Input: part model. Units: mm. Frame: model coordinates. A direction names the side the tool comes from. Give positions to 0.01 mm unless a question says otherwise; leave off trailing zeros. Write each loop counter-clockwise with the first axis right and the second up, starting at its lowest first coordinate (ties: lowest second). Pieces come first, ordered by that corner, then holes.
Autodesk Inventor part; units mm, degrees
ref_plane "Work Plane1" through (72.225, 0, 0) normal (1, 0, 0) x (0, 0, -1)
ref_plane "YZ Plane" through (0, 0, 0) normal (1, 0, 0) x (0, 1, 0)
ref_plane "XZ Plane" through (0, 0, 0) normal (0, 1, 0) x (-1, 0, 0)
sketch "Sketch1" plane through (0, 0, 0) normal (1, 0, 0) x (0, 1, 0)
  circle A0 centre (0, 0) radius 10
  arc A1 (-9.7398, 12.694) -> (5.3275, -15.087) centre (0, 0) ccw
  line L0 (0, 0) -> (0, 61.6) construction
  line L1 (0, 0) -> (54, 0) construction
  line L2 (0, 61.6) -> (54, 61.6) construction
  line L3 (54, 0) -> (54, 61.6) construction
  line L4 (54, 61.6) -> (54, 2.1)
  line L5 (54, 61.6) -> (-9.7398, 12.694)
  line L6 (54, 2.1) -> (5.3275, -15.087)
  dimension "d0" = 20
  dimension "d2" = 32
  dimension "d3" = 61.6
  dimension "d4" = 54
  dimension "d5" = 59.5
extrude "Extrusion1" add sketch "Sketch1" along normal blind 144.45
sketch "Sketch2" plane through (0, 0, 0) normal (0, 0, 1) x (1, 0, 0)
  line L0 (0, 54) -> (144.45, 54)
  line L1 (0, -9.7398) -> (0, 54)
  line L2 (0, -9.7398) -> (144.45, -9.7398)
  line L3 (144.45, 54) -> (144.45, -9.7398)
  line L4 (0, 54) -> (144.45, 54)
  line L5 (72.225, 54) -> (72.225, -21.6932)
  line L6 (39.225, 48) -> (105.225, 48)
  line L7 (105.225, 48) -> (105.225, -39.8615)
  line L8 (105.225, -39.8615) -> (39.225, -39.8615)
  line L9 (39.225, -39.8615) -> (39.225, 48)
  line L10 (72.225, 48) -> (72.225, -39.8615)
  point P0 (0, 0)
  dimension "d8" = 66
  dimension "d10" = 6
extrude "Extrusion2" cut sketch "Sketch2" along normal mid plane 144.45 contours L6 L7 L2 L5 | L5 L2 L9 L6 | L2 L5 L10 L8 L9 | L2 L7 L8 L10 L5
ref_plane "Work Plane1" through (72.225, 0, 0) normal (1, 0, 0) x (0, 0, -1)
sketch "Sketch3" plane through (0, 0, 0) normal (0, 0, 1) x (1, 0, 0)
  line L0 (0, 54) -> (144.45, 54)
  line L1 (144.45, 54) -> (144.45, -9.7398)
  line L2 (105.225, 48) -> (105.225, -9.7398)
  line L3 (105.225, -9.7398) -> (144.45, -9.7398)
  line L4 (144.45, 54) -> (144.45, -9.7398)
  line L5 (0, 54) -> (144.45, 54)
  line L6 (0, -9.7398) -> (0, 54)
  line L7 (0, -9.7398) -> (39.225, -9.7398)
  line L8 (39.225, -9.7398) -> (39.225, 48)
  line L9 (39.225, 48) -> (105.225, 48)
  line L10 (144.45, 48) -> (109.925, 48)
  line L11 (109.925, 48) -> (109.925, -25.7164)
  line L12 (109.925, -25.7164) -> (144.45, -25.7164)
  line L13 (144.45, -25.7164) -> (144.45, 48)
  line L14 (39.225, 48) -> (105.225, 48)
  point P0 (0, 0)
  dimension "d14" = 34.525
extrude "Extrusion3" cut sketch "Sketch3" along normal through all both and the other way through all contours L1 L3 L11 L10 | L13 L12 L11 L3
mirror "Mirror1" about plane through (72.225, 0, 0) normal (1, 0, 0) of "Extrusion3"
move or copy body "Move Body1" bodies to move or copy 1 copy no translate (-72.225, 0, 0)
move or copy body "Move Body2" bodies to move or copy 1 copy no rotation origin (0, 0, 0) rotation axis (1, 0, 0) rotation angle 90
move or copy body "Move Body4" bodies to move or copy 1 copy no rotation origin (0, 0, 0) rotation axis (0, 0, 1) rotation angle 90
properties part number "Head_v2"
Q1. Section B-B, the plane z = 0. Return the cut outline in (x, y).
Q2. Section D-D, the plane y = -22.5. Return the cut outline in (x, z), then the cut area to 3 significant figures.
Q3. Material intervals for line 1 along Y through (x, z) = (10.5, -5); line 2 along Z through (x, y) = (18, -44.5); line 3 along Z through (x, y) = (4, -37.5), sorted ascending.
Q4. Section C-C, the plane z = 43. Return the cut outline in (x, y), then the cut area to 3 significant figures.
Q5. Pin query (flat end, axial travel): pin 1 (12 mm diameter, centred on x = 1, z = 12, fed in from +Y); pin 2 (2 mm diameter, centred on x = 39.5, y = 18, fed in from -Z); pin 3 (4 mm diameter, centred on y = 32.5, z = 45.5, fed in from +X). Return the tip coordinate at first contact, or that it passes through.
Q6. Access query for faces 1 (the flat face through (12, -37.7, 23)), 2 (the flat face through (12, 37.7, 24)), 3 (the flat face through (12, 33, 24)), 4 (the cylindrical face through (9.76, -35.38, -2.17)), 5 (the flat face through (32, -1, 54)). Directions: +Z, -Z, +X, -X, +Y, -Y. A direction counts if a zero-diameter tool reaches every point of the face in a straight line with its end or side. Return the directions, or none.
Q7. Mould query, pull axis Y, two halves, no side actions, for faces 6 (the flat face through (31, 72.225, 51)), 7 (the flat face through (28, 0, 48)), 8 (the flat face through (28, 55, 48)). Classes: +Y half, -Y half, draft (parallel to the pull), parting line (faces both ways), or undercut.
Q8. Section A-A, the plane x = 6. Return the cut outline in (y, z) (3 decimals), then the cut area to 3 significant figures.
Solutions:
1. outline: (-16, -37.7) - (-10, -37.7) - (-10, -33) - (-16, -33) - close; (-16, 33) - (-10, 33) - (-10, 37.7) - (-16, 37.7) - close; (10, -37.7) - (20.17, -37.7) - (20.17, -33) - (10, -33) - close; (10, 33) - (20.17, 33) - (20.17, 37.7) - (10, 37.7) - close
2. outline: (-0.02, 48) - (57, 48) - (61.6, 54) - (2.1, 54) - close
2. area: 350 mm2
3. line 1: y = -37.7 to -33, 33 to 37.7
3. line 2: z = 48 to 54
3. line 3: z = -15.49 to -9.17, 9.17 to 54
4. outline: (-1.78, -37.7) - (53.16, -37.7) - (53.16, -33) - (-1.78, -33) - close; (-1.78, 33) - (53.16, 33) - (53.16, 37.7) - (-1.78, 37.7) - close
4. area: 516 mm2
5. pin 1: stops at y = 37.7
5. pin 2: stops at z = 48
5. pin 3: stops at x = 56.56
6. face 1: -Z, +X, -X, -Y
6. face 2: -Z, +X, -X, +Y
6. face 3: -Z, +X, -X
6. face 4: +Y, -Y
6. face 5: +Z, +X, -X, +Y, -Y
7. face 6: +Y half
7. face 7: undercut
7. face 8: draft
8. outline: (-72.225, 48) - (-37.7, 48) - (-37.7, 8) - (-33, 8) - (-33, 48) - (33, 48) - (33, 8) - (37.7, 8) - (37.7, 48) - (72.225, 48) - (72.225, 54) - (-72.225, 54) - close; (-37.7, -14.832) - (-33, -14.832) - (-33, -8) - (-37.7, -8) - close; (33, -14.832) - (37.7, -14.832) - (37.7, -8) - (33, -8) - close
8. area: 1,310 mm2
